```python
from build123d import *

# Parameters (mm, degrees)
BOSS_EXTRUDE1_DEPTH = 2
SKETCH10_W          = 280
SKETCH10_H          = 7
BOSS_EXTRUDE3_DEPTH = 2
SKETCH3_W           = 222
SKETCH3_H           = 13
BOSS_EXTRUDE4_DEPTH = 12.5
CHAMFER1_SIZE       = 5
FILLET1_R           = 1


with BuildPart() as part:
    # Sketch1 → Boss-Extrude1 (new body)
    with BuildSketch(Plane.XY):
        with BuildLine():
            Line((21.213203436, 24), (0, 2.786796564))
            Line((0, 2.786796564), (0, 0))
            Line((0, 0), (42, 0))
            Line((42, 0), (42, 11))
            ThreePointArc((42, 11), (43.171572875, 13.828427125), (46, 15))
            Line((46, 15), (262, 15))
            ThreePointArc((262, 15), (264.828427125, 13.828427125), (266, 11))
            Line((266, 11), (266, 0))
            Line((266, 0), (280, 0))
            Line((280, 0), (280, 2.786796564))
            Line((280, 2.786796564), (258.786796564, 24))
            Line((258.786796564, 24), (21.213203436, 24))
        make_face()
        with BuildLine():
            Line((42, 11), (42, 0))
            Line((42, 0), (266, 0))
            Line((266, 0), (266, 11))
            ThreePointArc((266, 11), (264.828427125, 13.828427125), (262, 15))
            Line((262, 15), (46, 15))
            ThreePointArc((46, 15), (43.171572875, 13.828427125), (42, 11))
        make_face()
    extrude(amount=BOSS_EXTRUDE1_DEPTH)

    # Sketch10 → Boss-Extrude3 (add)
    with BuildSketch(Plane.XZ):
        with Locations((140, 3.5)):
            Rectangle(SKETCH10_W, SKETCH10_H)
    extrude(amount=BOSS_EXTRUDE3_DEPTH)

    # Sketch3 → Boss-Extrude4 (add)
    with BuildSketch(Plane.XY.offset(2)):
        with Locations((154, 4.5)):
            Rectangle(SKETCH3_W, SKETCH3_H)
    extrude(amount=BOSS_EXTRUDE4_DEPTH)

    # Chamfer1
    chamfer1_edges = [part.edges().sort_by_distance(p)[0] for p in [
        (43, -1, 7),
        (0, -1, 7),
        (280, -1, 7),
        (265, -1, 7),
    ]]
    chamfer(chamfer1_edges, length=CHAMFER1_SIZE)

    # Fillet1
    fillet1_edges = [part.edges().sort_by_distance(p)[0] for p in [
        (0, 2.786796564, 1),
        (21.213203436, 24, 1),
        (258.786796564, 24, 1),
        (280, 2.786796564, 1),
        (280, -2, 1),
        (43, 4.5, 14.5),
        (154, -2, 14.5),
        (265, 4.5, 14.5),
        (0, -2, 1),
    ]]
    fillet(fillet1_edges, radius=FILLET1_R)


solid = part.part
```
Here's how the part is built. I have some questions about the finished solid (model axes, mm). A direction names the side the tool comes from. Round coordinates to 2 decimals unless told otherwise and drop trailing zeros. Order: outer loops, then holes, each group sorted by start corner. A loop starts at its lowest first (then second) coordinate and runs counter-clockwise, first axis right, second up. Notation, with made-up numbers: (19, 60.5) -> (44, 60.5) arc R25 ccw to (44, 85.5) -> close; hole circle Ø8 at (-40, 46.5). An arc over 180 degrees is marked (long way). Use a Markdown table: item, result. Add a question column.
(1) Suppose I cut it at B-B, the plane z = 9.5. Please give me the cut outline in (x, y).
(2) I need wall thicknesses on line 1 along Y through (x, z) = (50.5, 12.5); line 2 along Y through (x, z) = (15, 5.5); line 3 along Z through (x, y) = (32.5, 15). Which ranges of each line are inside material? Lowest first, please.
(3) For pin 1 Ø1.5 at (x, z) = (113.5, 6.5) entering from +Y; pin 2 Ø3 at (x, z) = (16, 9.5) entering from +Y; pin 3 Ø6 at (y, z) = (2.5, 9) entering from -X; pin 4 Ø1 at (x, y) = (25.5, -1) entering from +Z, each with a flat end and sliding along its axis, tell me the tip position at first contact or that it passes through.
(4) Suppose I cut it at C-C, the plane y = 5.5. Please give me the cut outline in (x, z).
(5) For faces 1 (the face through (43, 4, 8)), 2 (the face through (152, 5, 14.5)), 3 (the face through (271, 0, 5)), 4 (the face through (152, 11, 8)), which set-ups out of +Z, -Z, +X, -X, +Y, -Y let a thin tool reach every point of the face, with its end or its side?
(6) Suppose I cut it at D-D, the plane y = 20.5. Please give me the cut outline in (x, z).
(7) Suppose I cut it at A-A, the plane x = 75. Please give me the cut outline in (y, z).
Verdict:
| question | item | result |
|---|---|---|
| 1 | outline | (40.5, -2) -> (267.5, -2) -> (267.5, 0) -> (265, 0) -> (265, 11) -> (43, 11) -> (43, 0) -> (40.5, 0) -> close |
| 2 | line 1 | -2 to 11 |
| 2 | line 2 | -2 to 0 |
| 2 | line 3 | 0 to 2 |
| 3 | pin 1 | y = 11 |
| 3 | pin 2 | through |
| 3 | pin 3 | x = 38.34 |
| 3 | pin 4 | z = 7 |
| 4 | outline | (2.71, 0) -> (277.29, 0) -> (277.29, 2) -> (265, 2) -> (265, 13.5) arc R1 ccw to (264, 14.5) -> (44, 14.5) arc R1 ccw to (43, 13.5) -> (43, 2) -> (2.71, 2) -> close |
| 5 | face 1 | +Z, -X, +Y |
| 5 | face 2 | +Z, +X, -X, +Y, -Y |
| 5 | face 3 | +Z, +X, +Y |
| 5 | face 4 | +Z, +X, -X, +Y |
| 6 | outline | (17.71, 0) -> (262.29, 0) -> (262.29, 2) -> (17.71, 2) -> close |
| 7 | outline | (-2, 0) -> (24, 0) -> (24, 2) -> (11, 2) -> (11, 14.5) -> (-1, 14.5) arc R1 ccw to (-2, 13.5) -> close |
